```python
from build123d import *

# Parameters (mm, degrees)
F0_W     = 76.2
F0_H     = 171.45
F1_DEPTH = 22.225
F3_DEPTH = 22.226


with BuildPart() as f1:
    # F0 (on Front) → F1 (new body)
    with BuildSketch(Plane.XZ):
        with Locations((38.1, 85.725)):
            Rectangle(F0_W, F0_H)
    extrude(amount=F1_DEPTH)

    # F2 (on Front) → F3 (cut, through all)
    with BuildSketch(Plane.XZ):
        Polygon((28.575, 171.45), (23.033685, 149.225), (53.166315, 149.225), (47.625, 171.45), align=None)
        Polygon((76.2, 149.225), (76.2, 171.45), (70.658685, 149.225), align=None)
        Polygon((5.541315, 149.225), (0, 171.45), (0, 149.225), align=None)
        Polygon((70.658685, 22.225), (76.2, 0), (76.2, 22.225), align=None)
        Polygon((53.166315, 22.225), (23.033685, 22.225), (28.575, 0), (47.625, 0), align=None)
        Polygon((0, 22.225), (0, 0), (5.541315, 22.225), align=None)
    extrude(amount=F3_DEPTH, mode=Mode.SUBTRACT)


solid = f1.part
```
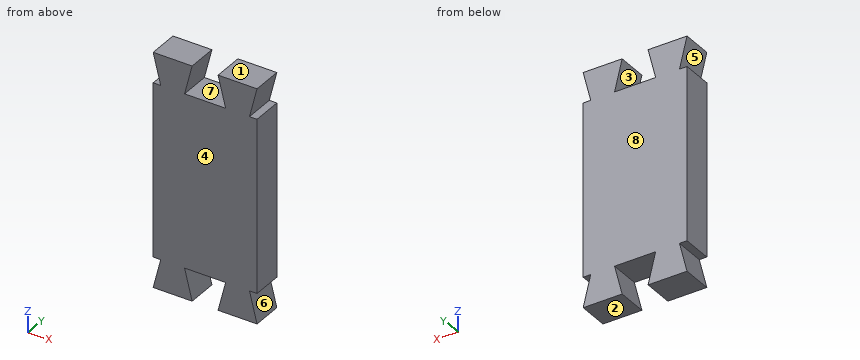
Geometry check sheet. Reference: the model listing, model coordinates, mm. Face numbers are marked on the shaded views. A direction names the side the tool comes from. Coordinates: 2 decimals unless noted, no trailing zeros. Write each loop counter-clockwise with the first axis right and the second up, starting at its lowest first coordinate (ties: lowest second). Pieces come first, ordered by that corner, then holes. Notation, with made-up numbers: M 65.25,48.5 L 104.25,48.5 A22 ccw 104.25,69.5 Z; hole C -15,34.25 d1. An arc over 180 degrees is marked long. One line per item, written item: value. Start each with the question number.
(1) Release check for a two-part mould opening along Z. For the marked faces 1, 2, 3 and 4 record: released by +Z, released by -Z, zero draft, split by the parting line, or undercut.
(2) Tool access check on the marked faces 5, 6, 7 and 8. Record the directions out of +Z, -Z, +X, -X, +Y, -Y that give a thin tool (end or side, any length) a straight path to the whole face; none if there is none.
(3) Scan lines: line 1 along Z through (x, y) = (29.5, -4) (3 decimals); line 2 along X through (y, z) = (-0.75, 163); line 3 along X through (y, z) = (-13.25, 155.5). Record each from-to range of solid material in increasing order. Write a range as [from, to].
(4) Depth check by flat-ended pin: pin 1 (8 mm diameter, centred on x = 31.5, z = 32, fed in from +Y); pin 2 (6.5 mm diameter, centred on x = 41.5, y = -11, fed in from +Z) (3 decimals). Enter the tip coordinate at first touch or a pass-through.
(5) Sectioned sample at A-A, the plane y = -14.5. Enter the section's corners in (x, z) (3 decimals), and give its area (3 significant figures).
Filled sheet:
1. face 1: released by +Z
1. face 2: released by -Z
1. face 3: undercut
1. face 4: zero draft
2. face 5: -X, +Y, -Y
2. face 6: +X, +Y, -Y
2. face 7: +Y, -Y
2. face 8: +Z, -Z, +X, -X, +Y
3. line 1: [22.225, 149.225]
3. line 2: [2.11, 26.47], [49.73, 74.09]
3. line 3: [3.98, 24.6], [51.6, 72.22]
4. pin 1: y = 0
4. pin 2: z = 149.225
5. outline: M 0,0 L 28.575,0 L 23.034,22.225 L 53.166,22.225 L 47.625,0 L 76.2,0 L 70.659,22.225 L 76.2,22.225 L 76.2,149.225 L 70.659,149.225 L 76.2,171.45 L 47.625,171.45 L 53.166,149.225 L 23.034,149.225 L 28.575,171.45 L 0,171.45 L 5.541,149.225 L 0,149.225 L 0,22.225 L 5.541,22.225 Z
5. area: 11,700 mm²
